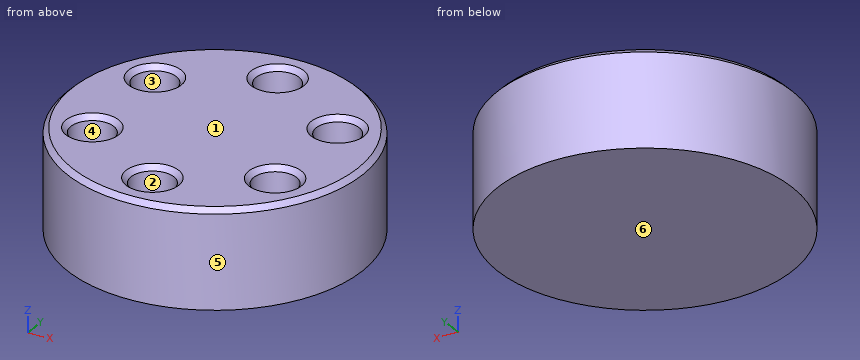
```python
from build123d import *

# Parameters (mm, degrees)
F0_R     = 38.1
F1_DEPTH = 25.4
F2_R     = 5.551213
F3_DEPTH = 19.05
F4_SIZE  = 1.27


with BuildPart() as f1:
    # F0 (on Top) → F1 (new body)
    with BuildSketch(Plane.XY):
        Circle(F0_R)
    extrude(amount=F1_DEPTH)

    # F2 (on face) → F3 (cut)
    with BuildSketch(Plane.XY.offset(25.4)):
        with Locations((0, 27.166931)):
            Circle(F2_R)
        with Locations((-23.527252, 13.583465)):
            Circle(F2_R)
        with Locations((-23.527252, -13.583465)):
            Circle(F2_R)
        with Locations((0, -27.166931)):
            Circle(F2_R)
        with Locations((23.527252, -13.583465)):
            Circle(F2_R)
        with Locations((23.527252, 13.583465)):
            Circle(F2_R)
    extrude(amount=-F3_DEPTH, mode=Mode.SUBTRACT)

    # F4
    f4_edges = [f1.edges().sort_by_distance(p)[0] for p in [
        (-5.551213, 27.166931, 25.4),
        (-38.1, 0, 25.4),
        (-29.078465, -13.583465, 25.4),
        (-5.551213, -27.166931, 25.4),
        (17.976039, -13.583465, 25.4),
        (-29.078465, 13.583465, 25.4),
        (17.976039, 13.583465, 25.4),
    ]]
    chamfer(f4_edges, length=F4_SIZE)


solid = f1.part
```
Could you check a few things on this model? Use its own coordinates, in mm. Face numbers are marked on the shaded views. A direction names the side the tool comes from. Round coordinates to 2 decimals unless told otherwise and drop trailing zeros. Loops run counter-clockwise (first coordinate to the right, second up) from the corner with the lowest first, then second, coordinate; pieces in that order, holes last. Notation, with made-up numbers: (49, 64.5) -> (82, 64.5) arc R37 cw to (82, 103.5) -> close; hole circle Ø7 at (60, 6). An arc over 180 degrees is marked (long way). Put each result on its own line as item: value.
Q1. For pin 1 Ø9 at (x, y) = (-1.5, -28) entering from +Z; pin 2 Ø10 at (y, z) = (-24, 15.5) entering from -X; pin 3 Ø4 at (y, z) = (-3.5, 20) entering from +X, each with a flat end and sliding along its axis, tell me the tip position at first contact or that it passes through.
Checks:
pin 1: z = 24.79
pin 2: x = -33.02
pin 3: x = 38.07
Q2. I want a section at A-A on x = 0. Write out the boundary of the cut face in (y, z).
Checks:
outline: (-38.1, 0) -> (38.1, 0) -> (38.1, 24.13) -> (36.83, 25.4) -> (33.99, 25.4) -> (32.72, 24.13) -> (32.72, 6.35) -> (21.62, 6.35) -> (21.62, 24.13) -> (20.35, 25.4) -> (-20.35, 25.4) -> (-21.62, 24.13) -> (-21.62, 6.35) -> (-32.72, 6.35) -> (-32.72, 24.13) -> (-33.99, 25.4) -> (-36.83, 25.4) -> (-38.1, 24.13) -> close
Q3. I want a section at C-C on z = 14.75. Write out the boundary of the cut face in (x, y).
Checks:
outline: circle Ø76.2 at (0, 0); hole circle Ø11.1 at (-23.53, -13.58); hole circle Ø11.1 at (-23.53, 13.58); hole circle Ø11.1 at (0, -27.17); hole circle Ø11.1 at (0, 27.17); hole circle Ø11.1 at (23.53, -13.58); hole circle Ø11.1 at (23.53, 13.58)
Q4. Thinking about a two-plate mould opening in X: for the marked faces 3, 4, 5 and 6, which applies, pulls with the +X half, pulls with the -X half, needs draft (parallel to the pull), parting line crosses it, or undercut?
Checks:
face 3: undercut
face 4: undercut
face 5: parting line crosses it
face 6: needs draft
Q5. I want a section at B-B on z = 4. Write out the boundary of the cut face in (x, y), and give its area (3 significant figures).
Checks:
outline: circle Ø76.2 at (0, 0)
area: 4,560 mm2
Q6. Which directions (+Z, -Z, +X, -X, +Y, -Y) give clear straight access to the entire face, cutting with the end or side of a thin tool? Please do the marked faces 1 and 2.
Checks:
face 1: +Z, +X, -X, +Y, -Y
face 2: +Z
Q7. Please list where these lines run through material, in increasing order: line 1 (Y direction, x = 0, z = 12.5); line 2 (Y direction, x = -4, z = 17.5); line 3 (X direction, y = -31, z = 23.75). Write a range as from..to.
Checks:
line 1: -38.1..-32.72, -21.62..21.62, 32.72..38.1
line 2: -37.89..-31.02, -23.32..23.32, 31.02..37.89
line 3: -22.15..-4.02, 4.02..22.15
